Autodesk Inventor part; units mm, degrees
ref_plane "YZ Plane" through (0, 0, 0) normal (1, 0, 0) x (0, 1, 0)
ref_plane "XZ Plane" through (0, 0, 0) normal (0, 1, 0) x (-1, 0, 0)
ref_plane "XY Plane" through (0, 0, 0) normal (0, 0, 1) x (1, 0, 0)
sketch "Sketch1" plane through (0, 0, 0) normal (0, 1, 0) x (-1, 0, 0)
  circle A0 centre (0, 0) radius 7.62
  dimension "d0" = 15.24
extrude "Extrusion1" add sketch "Sketch1" along normal blind 8.255
sketch "Sketch2" plane through (0, 8.255, 0) normal (0, 1, 0) x (1, 0, 0)
  circle A0 centre (0, 0) radius 7.62
  circle A1 centre (0, 0) radius 1.27
  dimension "d3" = 2.54
extrude "Extrusion2" add sketch "Sketch2" along normal blind 3.683 and the other way blind 11.938 contours A1
fillet "Fillet1" radius 1.5875 2 edges at (-1.27, 0, 0) (-1.27, 8.255, 0)
sketch "Sketch3" plane through (0, 8.255, 0) normal (0, 1, 0) x (1, 0, 0)
  circle A0 centre (0, 0) radius 7.62
  circle A1 centre (0, 0) radius 2.8575
properties part number "X Pulley"
Could you check a few things on this model? Use its own coordinates, in mm. A direction names the side the tool comes from. Give positions to 0.01 mm unless a question says otherwise; leave off trailing zeros. Order: outer loops, then holes, each group sorted by start corner. A loop starts at its lowest first (then second) coordinate and runs counter-clockwise, first axis right, second up. Notation, with made-up numbers: (67, 38) - (88, 38) arc R9 cw to (88, 43) - close; hole circle Ø6 at (0.25, -35.5). An arc over 180 degrees is marked (long way). Return JSON: item names as keys, results as strings. Group by question number.
Q1. Please list where these lines run through material, in increasing order: line 1 along Y through (x, z) = (-5.75, -1.75) (3 decimals); line 2 along X through (y, z) = (3, 5.25); line 3 along Z through (x, y) = (-6, 6.5). Write a range as [from, to].
Q2. Suppose I cut it at B-B, the plane z = 0. Please give me the cut outline in (x, y) (1 decimal).
Q3. Suppose I cut it at A-A, the plane x = 0. Please give me the cut outline in (y, z) (1 decimal).
Q4. Suppose I cut it at D-D, the plane z = -5.75. Please give me the cut outline in (x, y) (3 decimals).
Q5. Which directions (+Z, -Z, +X, -X, +Y, -Y) give clear straight access to the entire face, cutting with the end or side of a thin tool? Please do faces 1 (the face through (-0.17, -2.62, -1.26)), 2 (the face through (0.1, 8.255, -3.3)), 3 (the face through (1.65, 4.07, 7.44)).
Q6. Will these pins go through, and if not, where does the flat tip stop? pin 1 Ø3 at (x, y) = (3, 9) entering from +Z; pin 2 Ø6 at (x, z) = (-5, -3.5) entering from -Y; pin 3 Ø1 at (x, z) = (-6, -1) entering from +Y (3 decimals).
Q7. Suppose I cut it at C-C, the plane y = 6.25. Please give me the cut outline in (x, z), and give its area (3 significant figures).
Resolved:
{
 "1": {"line 1": "y = [0, 8.255]", "line 2": "x = [-5.52, 5.52]", "line 3": "z = [-4.7, 4.7]"},
 "2": {"outline": "(-7.6, 0) - (-2.9, 0) arc R1.6 cw to (-1.3, -1.6) - (-1.3, -3.7) - (1.3, -3.7) - (1.3, -1.6) arc R1.6 cw to (2.9, 0) - (7.6, 0) - (7.6, 8.3) - (2.9, 8.3) arc R1.6 cw to (1.3, 9.8) - (1.3, 11.9) - (-1.3, 11.9) - (-1.3, 9.8) arc R1.6 cw to (-2.9, 8.3) - (-7.6, 8.3) - close"},
 "3": {"outline": "(-3.7, -1.3) - (-1.6, -1.3) arc R1.6 cw to (0, -2.9) - (0, -7.6) - (8.3, -7.6) - (8.3, -2.9) arc R1.6 cw to (9.8, -1.3) - (11.9, -1.3) - (11.9, 1.3) - (9.8, 1.3) arc R1.6 cw to (8.3, 2.9) - (8.3, 7.6) - (0, 7.6) - (0, 2.9) arc R1.6 cw to (-1.6, 1.3) - (-3.7, 1.3) - close"},
 "4": {"outline": "(-5, 0) - (5, 0) - (5, 8.255) - (-5, 8.255) - close"},
 "5": {"face 1": "-Y", "face 2": "+Y", "face 3": "+Y, -Y"},
 "6": {"pin 1": "stops at z = 7.43", "pin 2": "stops at y = 0", "pin 3": "stops at y = 8.255"},
 "7": {"outline": "circle Ø15.24 at (0, 0)", "area": "182 mm2"}
}
